```python
from build123d import *

# Parameters (mm, degrees)
ESQUISSE1_W             = 13.74
ESQUISSE1_H             = 13.74
BOSS_EXTRU_1_DEPTH      = 20
ESQUISSE3_R             = 4.18
ENL_V_MAT_EXTRU_2_DEPTH = 10
ESQUISSE2_R             = 2.49
BOSS_EXTRU_4_DEPTH      = 24.8
ENL_V_START             = -24.8
ENL_V_MAT_EXTRU_4_DEPTH = 24.8
ESQUISSE6_R             = 5.5
ESQUISSE6_R_2           = 2.49
BOSS_EXTRU_5_DEPTH      = 24.8


with BuildPart() as part:
    # Esquisse1 → Boss.-Extru.1 (new body)
    with BuildSketch(Plane.XY):
        with Locations((-30.186071131, 8.6104)):
            Rectangle(ESQUISSE1_W, ESQUISSE1_H)
    extrude(amount=BOSS_EXTRU_1_DEPTH)

    # Esquisse3 → Enlèv. mat.-Extru.2 (cut)
    with BuildSketch(Plane.XY.offset(20)):
        with Locations((-30.186071131, 8.6104)):
            Circle(ESQUISSE3_R)
    extrude(amount=-ENL_V_MAT_EXTRU_2_DEPTH, mode=Mode.SUBTRACT)

    # Esquisse2 → Boss.-Extru.4 (add)
    with BuildSketch(Plane(origin=(0, 0, 0), x_dir=(-1, 0, 0), z_dir=(0, 0, -1))):
        with Locations(Location((30.186071131, 8.6104, 0), (0, 0, 180))):
            Circle(ESQUISSE2_R)
    extrude(amount=BOSS_EXTRU_4_DEPTH)

    # Esquisse5 → Enlèv. mat.-Extru.4 (cut)
    with BuildSketch(Plane(origin=(0, 0, -24.8), x_dir=(-1, 0, 0), z_dir=(0, 0, -1)).offset(ENL_V_START)):
        with BuildLine():
            Line((27.696071131, 8.6104), (29.625790006, 11.036546134))
            ThreePointArc((29.625790006, 11.036546134), (32.134814315, 7.0604), (27.696071131, 8.6104))
        make_face()
    extrude(amount=ENL_V_MAT_EXTRU_4_DEPTH, mode=Mode.SUBTRACT)

    # Esquisse6 → Boss.-Extru.5 (add)
    with BuildSketch(Plane(origin=(0, 0, 0), x_dir=(-1, 0, 0), z_dir=(0, 0, -1))):
        with Locations(Location((30.186071131, 8.6104, 0), (0, 0, 180))):
            Circle(ESQUISSE6_R)
        with Locations((30.186071131, 8.6104)):
            Circle(ESQUISSE6_R_2, mode=Mode.SUBTRACT)
    extrude(amount=BOSS_EXTRU_5_DEPTH)


solid = part.part
```
Model file for the job. Use its own axes, mm. A direction names the side the tool comes from. Coordinates: 2 decimals unless noted, no trailing zeros. Loops run counter-clockwise (first coordinate to the right, second up) from the corner with the lowest first, then second, coordinate; pieces in that order, holes last. Notation, with made-up numbers: (80, 45.25) - (103, 45.25) arc R18 cw to (103, 69.25) - close; hole circle Ø9 at (47.25, -9.5). An arc over 180 degrees is marked (long way). Answer as a JSON object with one key per item and string values. Group by question number.
(1) Cut at A-A (x = -31). Give the cut face in (y, z).
(2) Cut at B-B (y = 6.75). Give the cut face in (x, z), then the cut area to 3 significant figures.
(3) Cut at D-D (x = -33.5). Give the cut face in (y, z).
(4) Probe line 1 along Z through (x, y) = (-27.5, 11); line 2 along Z through (x, y) = (-36.5, 2.5); line 3 along X through (y, z) = (8.5, -13.5). List the from-to ranges inside material, lowest first.
(5) Two-plate mould, pull along Y, no slides. Class faces 4 (the face through (-28.65, 9.81, -12.23)), 5 (the face through (-30, 15.48, 10)), 6 (the face through (-28, 10, -24.8)), 7 (the face through (-30, 1.74, 10)): released by +Y, released by -Y, zero draft, split by the parting line, or undercut.
(6) Flat gauge pins, fed straight in: pin 1 (4 mm diameter, centred on x = -31, y = 8, fed in from +Z); pin 2 (2 mm diameter, centred on x = -26.5, z = -20, fed in from -Y). Where does each tip first touch, or does it go through?
(7) Cut at C-C (z = -6.5). Give the cut face in (x, y), then the cut area to 3 significant figures.
(8) Tool access for faces 1 (the face through (-26.2, 9.87, 15.07)), 2 (the face through (-23.316, 9, 10)), 3 (the face through (-32.08, 6.994, -12.226)): list every direction of +Z, -Z, +X, -X, +Y, -Y with a clear straight run to the whole face (end or side of a thin tool).
Geometry says:
{
 "1": {"outline": "(1.74, 0) - (3.17, 0) - (3.17, -24.8) - (6.26, -24.8) - (6.26, 0) - (10.96, 0) - (10.96, -24.8) - (14.05, -24.8) - (14.05, 0) - (15.48, 0) - (15.48, 20) - (12.71, 20) - (12.71, 10) - (4.51, 10) - (4.51, 20) - (1.74, 20) - close"},
 "2": {"outline": "(-37.06, 0) - (-35.36, 0) - (-35.36, -24.8) - (-31.84, -24.8) - (-31.84, 0) - (-28.53, 0) - (-28.53, -24.8) - (-25.01, -24.8) - (-25.01, 0) - (-23.32, 0) - (-23.32, 20) - (-26.44, 20) - (-26.44, 10) - (-33.93, 10) - (-33.93, 20) - (-37.06, 20) - close", "area": "375 mm^2"},
 "3": {"outline": "(1.74, 0) - (4.22, 0) - (4.22, -24.8) - (13, -24.8) - (13, 0) - (15.48, 0) - (15.48, 20) - (11.16, 20) - (11.16, 10) - (6.06, 10) - (6.06, 20) - (1.74, 20) - close"},
 "4": {"line 1": "z = -24.8 to 10", "line 2": "z = 0 to 20", "line 3": "x = -35.68 to -32.67, -27.7 to -24.69"},
 "5": {"face 4": "undercut", "face 5": "released by +Y", "face 6": "zero draft", "face 7": "released by -Y"},
 "6": {"pin 1": "stops at z = 10", "pin 2": "stops at y = 3.81"},
 "7": {"outline": "circle Ø11 at (-30.19, 8.61); hole (-29.63, 11.04) arc R2.49 ccw (long way) to (-27.7, 8.61) - close", "area": "76.7 mm^2"},
 "8": {"face 1": "+Z", "face 2": "+Z, -Z, +X, +Y, -Y", "face 3": "-Z"}
}
